Could you check a few things on this drawing? It's one solid part, dimensions in mm from its lowest x, y, z. Give positions to 0.01 mm unless a question says otherwise; leave off trailing zeros. Order: outer loops, then holes, each group sorted by start corner. A loop starts at its lowest first (then second) coordinate and runs counter-clockwise, first axis right, second up.
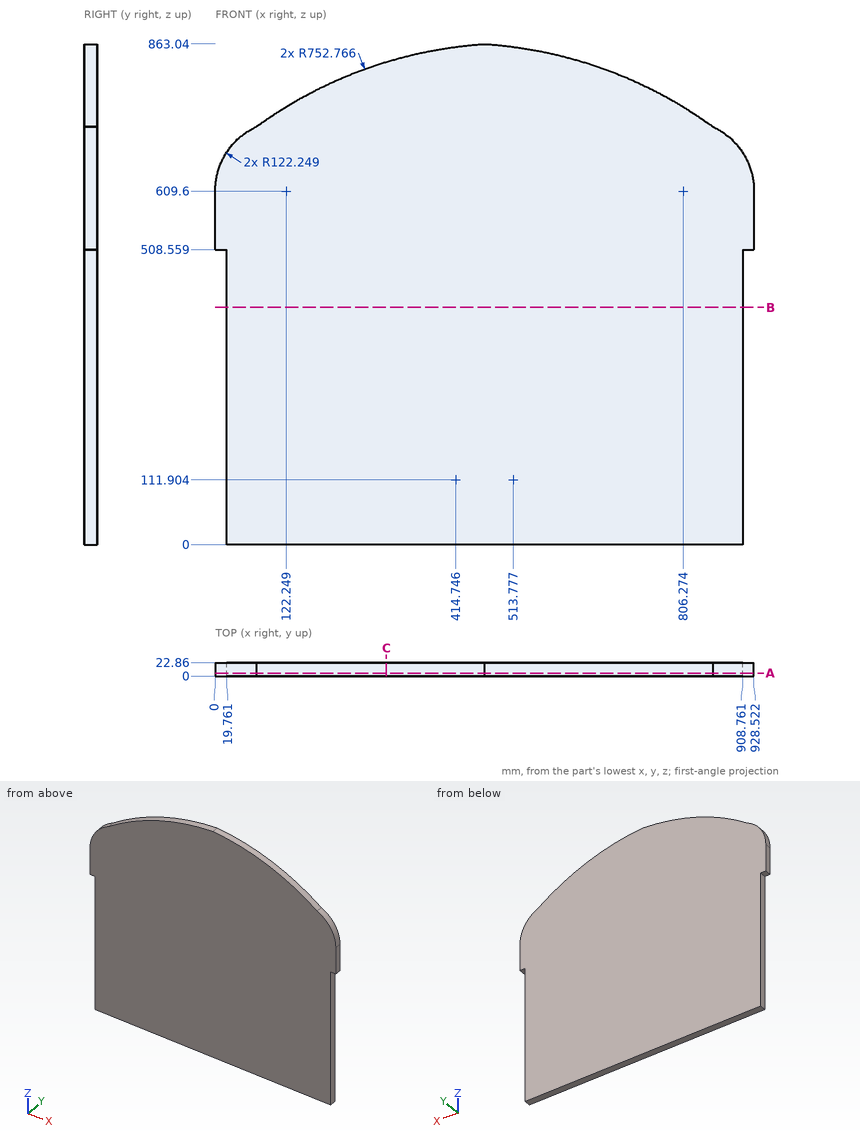
Item 1: Imagine slicing it at B-B on z = 409. List the corners of the cut face in (x, y) for me, then the cut area to 3 significant figures.
Findings:
outline: (19.76, 0) - (908.76, 0) - (908.76, 22.86) - (19.76, 22.86) - close
area: 20,300 mm2
Item 2: Imagine slicing it at C-C on x = 295. List the corners of the cut face in (y, z) for me, then the cut area to 3 significant figures.
Findings:
outline: (0, 0) - (22.86, 0) - (22.86, 832.18) - (0, 832.18) - close
area: 19,000 mm2
Item 3: Please list where these lines run through material, in increasing order: line 1 along X through (y, z) = (9.5, 341); line 2 along Z through (x, y) = (751, 10) (1 decimal); line 3 along Z through (x, y) = (104.5, 16) (1 decimal).
Findings:
line 1: x = 19.76 to 908.76
line 2: z = 0 to 785.4
line 3: z = 0 to 743.7
Item 4: Imagine slicing it at A-A on y = 4.75. List the corners of the cut face in (x, z) for me (1 decimal), then the cut area to 3 significant figures.
Findings:
outline: (0, 508.6) - (19.8, 508.6) - (19.8, 0) - (908.8, 0) - (908.8, 508.6) - (928.5, 508.6) - (928.5, 609.6) arc R122.2 ccw to (857.9, 720.4) arc R752.8 ccw to (464.3, 863) arc R752.8 ccw to (70.7, 720.4) arc R122.2 ccw to (0, 609.6) - close
area: 717,000 mm2
Item 5: For pin 1 (4 mm diameter, centred on y = 20.5, z = 293.5, fed in from +X); pin 2 (6 mm diameter, centred on y = 16, z = 183, fed in from -X); pin 3 (6 mm diameter, centred on x = 768.5, y = 14, fed in from +Z), each with a flat end and sliding along its axis, tell me the tip position at first contact or that it passes through.
Findings:
pin 1: stops at x = 908.76
pin 2: stops at x = 19.76
pin 3: stops at z = 777.96
